Autodesk Inventor part; units mm, degrees
ref_plane "YZ Plane" through (0, 0, 0) normal (1, 0, 0) x (0, 1, 0)
ref_plane "XZ Plane" through (0, 0, 0) normal (0, 1, 0) x (-1, 0, 0)
ref_plane "XY Plane" through (0, 0, 0) normal (0, 0, 1) x (1, 0, 0)
sketch "Sketch1" plane through (0, 0, 0) normal (0, 1, 0) x (-1, 0, 0)
  line L0 (0, -22) -> (0, 22)
  line L1 (0, 22) -> (1.5, 22)
  line L2 (1.5, 22) -> (1.5, 19)
  line L3 (1.5, 19) -> (3, 19)
  line L4 (3, 19) -> (3, -19)
  line L5 (3, -19) -> (1.5, -19)
  line L6 (1.5, -19) -> (1.5, -22)
  line L7 (1.5, -22) -> (0, -22)
  point P0 (0, 0)
  point P1 (0, 0)
  point P2 (3, 0)
  dimension "d1" = 6
  dimension "d2" = 3
  dimension "d3" = 3
  dimension "d4" = 44
revolve "Revolution1" add sketch "Sketch1" angle 360 about axis through (0, 0, -22) along (0, 0, 1)
thread "Thread1"
thread "Thread2"
equation "\"d4\" = L"
equation "\"L\" = 44"
properties part number "Shaft" material "Stainless Steel"
Model file for the job. Use its own axes, mm. A direction names the side the tool comes from. Coordinates: 2 decimals unless noted, no trailing zeros. Order: outer loops, then holes, each group sorted by start corner. A loop starts at its lowest first (then second) coordinate and runs counter-clockwise, first axis right, second up. Notation, with made-up numbers: (9.5, 51.5) -> (30.5, 51.5) arc R26 ccw to (30.5, 77.5) -> close; hole circle Ø5 at (83, -16.75). An arc over 180 degrees is marked (long way). Return JSON: item names as keys, results as strings.
Item 1: Pin check, flat tip, straight feed: P1, Ø1, axis at x = 2, y = -1.5, coming from the -Z side. Stop position of the tip, or through.
Model answer:
{"P1": "stops at z = -19"}
Item 2: Slice it at C-C (z = -18). Write the cut outline in (x, y), then the cut area to 3 significant figures.
Model answer:
{"outline": "circle Ø6 at (0, 0)", "area": "28.3 mm²"}
Item 3: Wall check: line 1 along X through (y, z) = (0.2, 16); line 2 along Z through (x, y) = (1.6, 0.9). Give the ranges that are in metal, low to high. Write a range as from..to.
Model answer:
{"line 1": "x = -2.99..2.99", "line 2": "z = -19..19"}
Item 4: 3-axis set-ups, long thin cutter, end or side, ignore diameter. For faces 1 (the face through (-1.3, 1.3, -19)), 2 (the face through (0, 0, -22)), 3 (the face through (-1.3, 1.3, 19)): which of +Z, -Z, +X, -X, +Y, -Y reach the whole face in a straight line?
Model answer:
{"face 1": "-Z", "face 2": "-Z, +X, -X, +Y, -Y", "face 3": "+Z"}
Item 5: Slice it at A-A (y = 0). Write the cut outline in (x, z).
Model answer:
{"outline": "(-3, -19) -> (-1.5, -19) -> (-1.5, -22) -> (1.5, -22) -> (1.5, -19) -> (3, -19) -> (3, 19) -> (1.5, 19) -> (1.5, 22) -> (-1.5, 22) -> (-1.5, 19) -> (-3, 19) -> close"}
Item 6: Slice it at D-D (y = -2.1). Write the cut outline in (x, z), then the cut area to 3 significant figures.
Model answer:
{"outline": "(-2.14, -19) -> (2.14, -19) -> (2.14, 19) -> (-2.14, 19) -> close", "area": "163 mm²"}
